The model under review builds one solid part; all positions refer to its coordinate system, in mm. A direction names the side the tool comes from. Coordinates: 2 decimals unless noted, no trailing zeros. Write each loop counter-clockwise with the first axis right and the second up, starting at its lowest first coordinate (ties: lowest second). Pieces come first, ordered by that corner, then holes. Notation, with made-up numbers: (5.5, 77) - (43.5, 77) arc R16 ccw to (43.5, 100) - close; hole circle Ø7 at (9.25, -28.75). An arc over 180 degrees is marked (long way). Put each result on its own line as item: value. Start each with the question number.
Item 1: Machinability: for faces 4 (the face through (-20, 1, -3)), 5 (the face through (10, 2, -53)), which of the approach directions +Z, -Z, +X, -X, +Y, -Y give a long, thin tool a straight path to every point of the face, cutting with its end or side? Answer none if there is none.
Item 2: For pin 1 (4 mm diameter, centred on x = -2.5, z = 30.5, fed in from -Y), flat-tipped, find the tip position at first contact; note if it passes through.
Item 3: To check wall thickness, follow L1, parallel to X at y = 1.85, z = 19; L2, parallel to X at y = 0.3, z = 22; L3, parallel to Z at x = 10.5, y = 1.9. State the ranges of each line that lie inside material, in increasing order. Write a range as [from, to].
Item 4: Consider section A-A on x = -4. Give the boundary of the cut face in (y, z), then the cut area to 3 significant figures.
Item 5: Consider section B-B on x = 10. Give the boundary of the cut face in (y, z).
Item 6: Mouldability with a two-part tool opening along Z and no side actions: class faces 1 (the face through (20, 1, -1)), 2 (the face through (-18.13, 2.87, -58.06)), 3 (the face through (-13, 2, -45)) as pulls with the +Z half, pulls with the -Z half, needs draft (parallel to the pull), parting line crosses it, or undercut.
Autodesk Inventor part; units mm, degrees
ref_plane "YZ Plane" through (0, 0, 0) normal (1, 0, 0) x (0, 1, 0)
ref_plane "XZ Plane" through (0, 0, 0) normal (0, 1, 0) x (-1, 0, 0)
ref_plane "XY Plane" through (0, 0, 0) normal (0, 0, 1) x (1, 0, 0)
sketch "Sketch1" plane through (0, 0, 0) normal (0, 1, 0) x (-1, 0, 0)
  line L0 (-20, 60) -> (20, 60)
  line L1 (20, 60) -> (20, -60)
  line L2 (20, -60) -> (-20, -60)
  line L3 (-20, -60) -> (-20, 60)
  line L4 (-20, 60) -> (20, -60) construction
  line L5 (20, 60) -> (-20, -60) construction
  point P0 (0, 0)
  dimension "d0" = 120
  dimension "d1" = 40
extrude "Extrusion1" add sketch "Sketch1" along normal blind 3
sketch "Sketch2" plane through (0, 3, 0) normal (0, 1, 0) x (1, 0, 0)
  line L0 (-10, -20) -> (-10, -10) construction
  line L1 (-7, -20) -> (-7, -10)
  line L2 (-13, -10) -> (-13, -20)
  arc A0 (-13, -20) -> (-7, -20) centre (-10, -20) ccw
  arc A1 (-7, -10) -> (-13, -10) centre (-10, -10) ccw
  line L3 (-32, 15) -> (32, 15) construction
  line L4 (20, 60) -> (-20, 60)
  line L5 (0, 84) -> (0, -84)
  line L6 (-10, 50) -> (-10, 40) construction
  line L7 (-7, 50) -> (-7, 40)
  line L8 (-13, 40) -> (-13, 50)
  arc A2 (-7, 50) -> (-13, 50) centre (-10, 50) ccw
  arc A3 (-13, 40) -> (-7, 40) centre (-10, 40) ccw
  line L9 (10, -20) -> (10, -10) construction
  line L10 (7, -20) -> (7, -10)
  line L11 (13, -10) -> (13, -20)
  arc A4 (7, -20) -> (13, -20) centre (10, -20) ccw
  arc A5 (13, -10) -> (7, -10) centre (10, -10) ccw
  line L12 (10, 50) -> (10, 40) construction
  line L13 (7, 50) -> (7, 40)
  line L14 (13, 40) -> (13, 50)
  arc A6 (13, 50) -> (7, 50) centre (10, 50) ccw
  arc A7 (7, 40) -> (13, 40) centre (10, 40) ccw
  point P0 (0, 0)
  point P1 (-10, -15)
  point P2 (-10, 45)
  point P3 (10, -15)
  point P4 (10, 45)
  dimension "d4" = 3
  dimension "d5" = 10
  dimension "d6" = 30
  dimension "d7" = 45
  dimension "d8" = 10
sketch "Sketch3" plane through (0, 3, 0) normal (0, 1, 0) x (1, 0, 0)
  circle A0 centre (-4, -51) radius 2.25
  line L0 (-20, -60) -> (20, -60)
  line L1 (20, -60) -> (20, 60)
  line L2 (-20, 60) -> (-20, -60)
  point P0 (0, 0)
  dimension "d9" = 4.5
  dimension "d10" = 9
  dimension "d16" = 16
extrude "Extrusion2" cut sketch "Sketch3" against normal blind 3
extrude "Extrusion3" cut sketch "Sketch2" against normal blind 3
chamfer "Chamfer1" distance 10 angle 45 1 edges at (-20, 1.5, 60)
fillet "Fillet1" radius 5 5 edges at (-10, 1.5, 60) (-20, 1.5, 50) (20, 1.5, 60) (20, 1.5, -60) (-20, 1.5, -60)
chamfer "Chamfer2" distance 0.75 angle 45 10 edges at (20, 3, 0) (18.5355, 3, -58.5355) (0, 3, -60) (-18.5355, 3, -58.5355) (-20, 3, -3.5355) (-19.6194, 3, 49.8423) (-15, 3, 55) (-9.8423, 3, 59.6194) (3.5355, 3, 60) (18.5355, 3, 58.5355)
properties part number "Rear"
Report:
1. face 4: +Z, -Z, -X, +Y, -Y
1. face 5: +Y, -Y
2. pin 1: y = 0
3. L1: [-20, -13], [-7, 7], [13, 20]
3. L2: [-20, -12.24], [-7.76, 7.76], [12.24, 20]
3. L3: [-60, -52.96], [-37.04, 7.04], [22.96, 60]
4. outline: (0, -60) - (2.25, -60) - (3, -59.25) - (3, 48.75) - (0, 48.75) - close; (0, 53.25) - (3, 53.25) - (3, 59.25) - (2.25, 60) - (0, 60) - close
4. area: 346 mm²
5. outline: (0, -60) - (2.25, -60) - (3, -59.25) - (3, -53) - (0, -53) - close; (0, -37) - (3, -37) - (3, 7) - (0, 7) - close; (0, 23) - (3, 23) - (3, 59.25) - (2.25, 60) - (0, 60) - close
6. face 1: needs draft
6. face 2: pulls with the -Z half
6. face 3: undercut
